Check sheet for the modelled part. Datum: model origin and axes. Units: mm. Face numbers are marked on the shaded views. Give positions to 0.01 mm unless a question says otherwise; leave off trailing zeros. Write each loop counter-clockwise with the first axis right and the second up, starting at its lowest first coordinate (ties: lowest second). Pieces come first, ordered by that corner, then holes. Notation, with made-up numbers: (-26.75, 19) -> (16.25, 19) arc R35 cw to (16.25, 53) -> close; hole circle Ø8 at (77.25, -22.75). An arc over 180 degrees is marked (long way). Use a Markdown table: item, result. Add a question column.
1. Cross-section at C-C (x = 68). Enter the section's corners in (y, z), then the cut area to 3 significant figures.
2. Release check for a two-part mould opening along Z. For the marked faces 1 and 2 record: released by +Z, released by -Z, zero draft, split by the parting line, or undercut.
3. Cross-section at B-B (z = 20). Enter the section's corners in (x, y), then the cut area to 3 significant figures.
4. Gauge pin test, flat ends, axial feed: P1, Ø0.5, axis at y = 6.5, z = 38.5, coming from the +X side; P2, Ø0.5, axis at x = -29.5, z = 38.5, coming from the -Y side; P3, Ø6, axis at x = 61.5, y = 1.5, coming from the -Z side; P4, Ø23, axis at x = 22, z = -19, coming from the +Y side. Record the tip position at first contact, or that the pin passes through.
5. Cross-section at A-A (x = -58). Enter the section's corners in (y, z).
6. Scan lines: probe 1 along X at (y, z) = (10.25, 33.5); probe 2 along Z at (x, y) = (-59.5, 3); probe 3 along Y at (x, z) = (48.5, 18.5). Record each from-to range of solid material in increasing order. Write a range as [from, to].
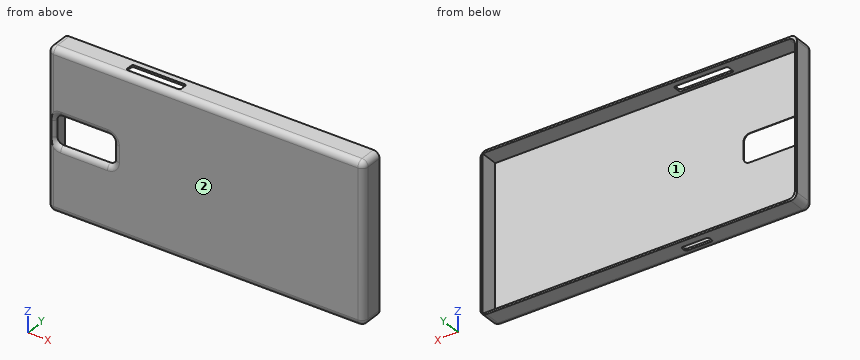
from build123d import *

# Parameters (mm, degrees)
SKETCH1_W           = 154.9
SKETCH1_H           = 77.9
BOSS_EXTRUDE1_DEPTH = 10.9
SKETCH8_W           = 152.9
SKETCH8_H           = 75.9
CUT_EXTRUDE3_DEPTH  = 8.9
FILLET6_R           = 2.99
FILLET7_R           = 2.99
FILLET8_R           = 2.99
FILLET9_R           = 2.99
FILLET10_R          = 2.99
FILLET11_R          = 2.99
FILLET12_R          = 2.99
FILLET13_R          = 2.99
SKETCH12_W          = 28.9
SKETCH12_H          = 13.9
CUT_EXTRUDE4_DEPTH  = 88.148235782
FILLET15_R          = 2.99
FILLET16_R          = 2.99
FILLET17_R          = 2.99
FILLET18_R          = 2.99
CUT_EXTRUDE8_REACH  = 112.389
SKETCH15_W          = 26.5
SKETCH15_H          = 4.5
CUT_EXTRUDE9_REACH  = 112.389
SKETCH16_W          = 13.5
SKETCH16_H          = 3.3
FILLET19_R          = 2.99
FILLET22_R          = 0.9
FILLET23_R          = 0.9
FILLET24_R          = 0.9
FILLET25_R          = 0.9
FILLET29_R          = 0.9
FILLET39_R          = 2.99
SKETCH6_W           = 152.9
SKETCH6_H           = 75.9
CUT_EXTRUDE2_DEPTH  = 8.9
FILLET4_R           = 2.99
FILLET5_R           = 2.99


with BuildPart() as part:
    # Sketch1 → Boss-Extrude1 (new body)
    with BuildSketch(Plane(origin=(0, 0, 0), x_dir=(1, 0, 0), z_dir=(0, 1, 0))):
        Rectangle(SKETCH1_W, SKETCH1_H)
    extrude(amount=BOSS_EXTRUDE1_DEPTH)

    # Sketch8 → Cut-Extrude3 (cut)
    with BuildSketch(Plane(origin=(0, 10.9, 0), x_dir=(1, 0, 0), z_dir=(0, 1, 0))):
        Rectangle(SKETCH8_W, SKETCH8_H)
    extrude(amount=-CUT_EXTRUDE3_DEPTH, mode=Mode.SUBTRACT)

    # Fillet6
    fillet6_edges = [part.edges().sort_by_distance(p)[0] for p in [
        (-76.45, 6.45, -37.95),
    ]]
    fillet(fillet6_edges, radius=FILLET6_R)

    # Fillet7
    fillet7_edges = [part.edges().sort_by_distance(p)[0] for p in [
        (-76.45, 6.45, 37.95),
    ]]
    fillet(fillet7_edges, radius=FILLET7_R)

    # Fillet8
    fillet8_edges = [part.edges().sort_by_distance(p)[0] for p in [
        (76.45, 6.45, -37.95),
    ]]
    fillet(fillet8_edges, radius=FILLET8_R)

    # Fillet9
    fillet9_edges = [part.edges().sort_by_distance(p)[0] for p in [
        (76.45, 6.45, 37.95),
    ]]
    fillet(fillet9_edges, radius=FILLET9_R)

    # Fillet10
    fillet10_edges = [part.edges().sort_by_distance(p)[0] for p in [
        (77.45, 5.45, 38.95),
    ]]
    fillet(fillet10_edges, radius=FILLET10_R)

    # Fillet11
    fillet11_edges = [part.edges().sort_by_distance(p)[0] for p in [
        (-77.45, 5.45, 38.95),
    ]]
    fillet(fillet11_edges, radius=FILLET11_R)

    # Fillet12
    fillet12_edges = [part.edges().sort_by_distance(p)[0] for p in [
        (-77.45, 5.45, -38.95),
    ]]
    fillet(fillet12_edges, radius=FILLET12_R)

    # Fillet13
    fillet13_edges = [part.edges().sort_by_distance(p)[0] for p in [
        (1.495, 0, -38.95),
        (77.45, 0, -1.495),
        (76.574249276, 0, 38.074249276),
        (0, 0, 38.95),
        (-76.574249276, 0, 38.074249276),
        (-77.45, 0, 0),
        (-76.574249276, 0, -38.074249276),
    ]]
    fillet(fillet13_edges, radius=FILLET13_R)

    # Sketch12 → Cut-Extrude4 (cut, through all)
    with BuildSketch(Plane(origin=(0, 2, 0), x_dir=(1, 0, 0), z_dir=(0, 1, 0))):
        with Locations((-59.543133303, -0.270064355)):
            Rectangle(SKETCH12_W, SKETCH12_H)
    extrude(amount=-CUT_EXTRUDE4_DEPTH, mode=Mode.SUBTRACT)

    # Fillet15
    fillet15_edges = [part.edges().sort_by_distance(p)[0] for p in [
        (-73.993133303, 1, -6.679935645),
    ]]
    fillet(fillet15_edges, radius=FILLET15_R)

    # Fillet16
    fillet16_edges = [part.edges().sort_by_distance(p)[0] for p in [
        (-73.993133303, 1, 7.220064355),
    ]]
    fillet(fillet16_edges, radius=FILLET16_R)

    # Fillet17
    fillet17_edges = [part.edges().sort_by_distance(p)[0] for p in [
        (-45.093133303, 1, 7.220064355),
    ]]
    fillet(fillet17_edges, radius=FILLET17_R)

    # Fillet18
    fillet18_edges = [part.edges().sort_by_distance(p)[0] for p in [
        (-45.093133303, 1, -6.679935645),
    ]]
    fillet(fillet18_edges, radius=FILLET18_R)

    # Sketch15 → Cut-Extrude8 (cut, up to next)
    with BuildSketch(Plane.XY.offset(38.95), mode=Mode.PRIVATE) as cut_extrude8_sk1:
        with Locations((-28.269520984, 5.746289853)):
            Rectangle(SKETCH15_W, SKETCH15_H)
    cut_extrude8_tool1 = extrude(cut_extrude8_sk1.sketch, amount=-CUT_EXTRUDE8_REACH, mode=Mode.PRIVATE) & part.part
    add(cut_extrude8_tool1.solids().sort_by_distance((-28.269521, 5.74629, 38.95))[0], mode=Mode.SUBTRACT)

    # Sketch16 → Cut-Extrude9 (cut, up to next)
    with BuildSketch(Plane(origin=(0, 0, -38.95), x_dir=(-1, 0, 0), z_dir=(0, 0, -1)), mode=Mode.PRIVATE) as cut_extrude9_sk1:
        with Locations((24.905722524, 5.653111576)):
            Rectangle(SKETCH16_W, SKETCH16_H)
    cut_extrude9_tool1 = extrude(cut_extrude9_sk1.sketch, amount=-CUT_EXTRUDE9_REACH, mode=Mode.PRIVATE) & part.part
    add(cut_extrude9_tool1.solids().sort_by_distance((-24.905723, 5.653112, -38.95))[0], mode=Mode.SUBTRACT)

    # Fillet19
    # the kernel refuses this fillet: 2.99 mm, written as the material it takes off along each edge
    with BuildSketch(Plane(origin=(-71.003133303, 0, 4.230064355), x_dir=(-1, 0, 0), z_dir=(0, 0, -1))) as fillet19_piece_1:
        with BuildLine():
            CenterArc((5.811347196, 2.99), FILLET19_R, 199.335777997, 70.664222003)
            Line((2.99, 2), (2.933573056, 1.9802))
            ThreePointArc((2.933573056, 1.9802), (2.9302, 1), (2.9302, 0))
            Line((2.9302, 0), (2.99, -0.0598))
            Line((2.99, -0.0598), (5.811347196, -0.0598))
            Line((5.811347196, -0.0598), (5.811347196, 0))
        make_face()
    revolve(axis=Axis((-71.003133303, 0, 4.230064355), (0, 1, 0)), revolution_arc=90, mode=Mode.SUBTRACT)
    with BuildSketch(Plane(origin=(-73.993133303, 0, -3.689935645), x_dir=(-1, 0, 0), z_dir=(0, 0, 1)), Plane(origin=(-45.093133303, 0, 4.230064355), x_dir=(1, 0, 0), z_dir=(0, 0, -1))) as fillet19_piece_2:
        with BuildLine():
            CenterArc((2.821347196, -2.99), FILLET19_R, 90, 70.664222003)
            Line((0, -2), (-0.056426944, -1.9802))
            ThreePointArc((-0.056426944, -1.9802), (-0.0598, -1), (-0.0598, 0))
            Line((-0.0598, 0), (0, 0.0598))
            Line((0, 0.0598), (2.821347196, 0.0598))
            Line((2.821347196, 0.0598), (2.821347196, 0))
        make_face()
    extrude(amount=7.92, mode=Mode.SUBTRACT)
    with BuildSketch(Plane(origin=(-71.003133303, 0, -3.689935645), x_dir=(0, 0, -1), z_dir=(1, 0, 0))) as fillet19_piece_3:
        with BuildLine():
            CenterArc((5.811347196, 2.99), FILLET19_R, 199.335777997, 70.664222003)
            Line((2.99, 2), (2.933573056, 1.9802))
            ThreePointArc((2.933573056, 1.9802), (2.9302, 1), (2.9302, 0))
            Line((2.9302, 0), (2.99, -0.0598))
            Line((2.99, -0.0598), (5.811347196, -0.0598))
            Line((5.811347196, -0.0598), (5.811347196, 0))
        make_face()
    revolve(axis=Axis((-71.003133303, 0, -3.689935645), (0, 1, 0)), revolution_arc=90, mode=Mode.SUBTRACT)
    with BuildSketch(Plane(origin=(-48.083133303, 0, -6.679935645), x_dir=(0, 0, -1), z_dir=(-1, 0, 0)), Plane(origin=(-71.003133303, 0, 7.220064355), x_dir=(0, 0, 1), z_dir=(1, 0, 0))) as fillet19_piece_4:
        with BuildLine():
            CenterArc((2.821347196, -2.99), FILLET19_R, 90, 70.664222003)
            Line((0, -2), (-0.056426944, -1.9802))
            ThreePointArc((-0.056426944, -1.9802), (-0.0598, -1), (-0.0598, 0))
            Line((-0.0598, 0), (0, 0.0598))
            Line((0, 0.0598), (2.821347196, 0.0598))
            Line((2.821347196, 0.0598), (2.821347196, 0))
        make_face()
    extrude(amount=22.92, mode=Mode.SUBTRACT)
    with BuildSketch(Plane(origin=(-48.083133303, 0, -3.689935645), x_dir=(1, 0, 0), z_dir=(0, 0, 1))) as fillet19_piece_5:
        with BuildLine():
            CenterArc((5.811347196, 2.99), FILLET19_R, 199.335777997, 70.664222003)
            Line((2.99, 2), (2.933573056, 1.9802))
            ThreePointArc((2.933573056, 1.9802), (2.9302, 1), (2.9302, 0))
            Line((2.9302, 0), (2.99, -0.0598))
            Line((2.99, -0.0598), (5.811347196, -0.0598))
            Line((5.811347196, -0.0598), (5.811347196, 0))
        make_face()
    revolve(axis=Axis((-48.083133303, 0, -3.689935645), (0, 1, 0)), revolution_arc=90, mode=Mode.SUBTRACT)
    with BuildSketch(Plane(origin=(-48.083133303, 0, 4.230064355), x_dir=(0, 0, 1), z_dir=(-1, 0, 0))) as fillet19_piece_6:
        with BuildLine():
            CenterArc((5.811347196, 2.99), FILLET19_R, 199.335777997, 70.664222003)
            Line((2.99, 2), (2.933573056, 1.9802))
            ThreePointArc((2.933573056, 1.9802), (2.9302, 1), (2.9302, 0))
            Line((2.9302, 0), (2.99, -0.0598))
            Line((2.99, -0.0598), (5.811347196, -0.0598))
            Line((5.811347196, -0.0598), (5.811347196, 0))
        make_face()
    revolve(axis=Axis((-48.083133303, 0, 4.230064355), (0, 1, 0)), revolution_arc=90, mode=Mode.SUBTRACT)

    # Fillet22
    fillet22_edges = [part.edges().sort_by_distance(p)[0] for p in [
        (-15.019520984, 7.996289853, 38.45),
    ]]
    fillet(fillet22_edges, radius=FILLET22_R)

    # Fillet23
    fillet23_edges = [part.edges().sort_by_distance(p)[0] for p in [
        (-41.519520984, 7.996289853, 38.45),
    ]]
    fillet(fillet23_edges, radius=FILLET23_R)

    # Fillet24
    fillet24_edges = [part.edges().sort_by_distance(p)[0] for p in [
        (-15.019520984, 3.496289853, 38.45),
    ]]
    fillet(fillet24_edges, radius=FILLET24_R)

    # Fillet25
    fillet25_edges = [part.edges().sort_by_distance(p)[0] for p in [
        (-41.519520984, 3.496289853, 38.45),
    ]]
    fillet(fillet25_edges, radius=FILLET25_R)

    # Fillet29
    fillet29_edges = [part.edges().sort_by_distance(p)[0] for p in [
        (-31.655722524, 7.303111576, -38.45),
        (-31.655722524, 4.003111576, -38.45),
        (-18.155722524, 4.003111576, -38.45),
        (-18.155722524, 7.303111576, -38.45),
    ]]
    fillet(fillet29_edges, radius=FILLET29_R)

    # Fillet39
    # the kernel refuses this fillet: 2.99 mm, written as the material it takes off along each edge
    with BuildSketch(Plane(origin=(74.46, 2.99, -35.96), x_dir=(1, 0, 0), z_dir=(0, 0, -1))) as fillet39_piece_1_section:
        Polygon((0, 0), (FILLET39_R, 0), (FILLET39_R, FILLET39_R), (0, FILLET39_R), align=None)
    fillet39_piece_1 = extrude(amount=FILLET39_R, mode=Mode.PRIVATE)
    fillet39_piece_1 = fillet39_piece_1 - Plane(origin=(74.46, 2.99, -35.96), x_dir=(-0.7071067811865475, 0.7071067811865475, 0), z_dir=(0, 0, -1)) * Sphere(FILLET39_R, mode=Mode.PRIVATE)
    add(fillet39_piece_1, mode=Mode.SUBTRACT)
    with BuildSketch(Plane(origin=(77.45, 2.99, -38.95), x_dir=(-1, 0, 0), z_dir=(0, 1, 0))) as fillet39_piece_2:
        with BuildLine():
            CenterArc((FILLET39_R, FILLET39_R), FILLET39_R, 180, 90)
            Line((0, FILLET39_R), (0, 0))
            Line((0, 0), (FILLET39_R, 0))
        make_face()
    extrude(amount=15.385, mode=Mode.SUBTRACT)

    # Sketch6 → Cut-Extrude2 (cut)
    with BuildSketch(Plane(origin=(0, 10.9, 0), x_dir=(1, 0, 0), z_dir=(0, 1, 0))):
        Rectangle(SKETCH6_W, SKETCH6_H)
    extrude(amount=-CUT_EXTRUDE2_DEPTH, mode=Mode.SUBTRACT)

    # Fillet4
    fillet4_edges = [part.edges().sort_by_distance(p)[0] for p in [
        (-76.45, 6.45, -37.95),
    ]]
    fillet(fillet4_edges, radius=FILLET4_R)

    # Fillet5
    fillet5_edges = [part.edges().sort_by_distance(p)[0] for p in [
        (-76.45, 6.45, 37.95),
    ]]
    fillet(fillet5_edges, radius=FILLET5_R)


solid = part.part
Worked answers:
| question | item | result |
|---|---|---|
| 1 | outline | (0, -35.96) arc R2.99 ccw to (2.99, -38.95) -> (10.9, -38.95) -> (10.9, -37.95) -> (2, -37.95) -> (2, 37.95) -> (10.9, 37.95) -> (10.9, 38.95) -> (2.99, 38.95) arc R2.99 ccw to (0, 35.96) -> close |
| 1 | area | 170 mm² |
| 2 | face 1 | undercut |
| 2 | face 2 | zero draft |
| 3 | outline | (-77.45, 2.99) arc R2.99 ccw to (-74.46, 0) -> (74.46, 0) arc R2.99 ccw to (77.45, 2.99) -> (77.45, 10.9) -> (76.45, 10.9) -> (76.45, 2) -> (-76.45, 2) -> (-76.45, 10.9) -> (-77.45, 10.9) -> close |
| 3 | area | 324 mm² |
| 4 | P1 | stops at x = 76.38 |
| 4 | P2 | stops at y = 1.07 |
| 4 | P3 | stops at z = -38.95 |
| 4 | P4 | stops at y = 2 |
| 5 | outline | (0, -35.96) arc R2.99 ccw to (2.99, -38.95) -> (10.9, -38.95) -> (10.9, -37.95) -> (2, -37.95) -> (2, -6.68) arc R2.99 ccw to (0, -9.5) -> close; (0, 10.04) arc R2.99 ccw to (2, 7.22) -> (2, 37.95) -> (10.9, 37.95) -> (10.9, 38.95) -> (2.99, 38.95) arc R2.99 ccw to (0, 35.96) -> close |
| 6 | probe 1 | x = [-77.45, -76.45], [76.45, 77.45] |
| 6 | probe 2 | z = [-38.95, -37.95], [37.95, 38.95] |
| 6 | probe 3 | y = [0, 2] |
